For this review, take the finished solid that the model builds, in its own axes (mm). Face numbers are marked on the shaded views. A direction names the side the tool comes from. Coordinates: 2 decimals unless noted, no trailing zeros. Order: outer loops, then holes, each group sorted by start corner. A loop starts at its lowest first (then second) coordinate and runs counter-clockwise, first axis right, second up. Notation, with made-up numbers: (85.25, 70.5) -> (123.25, 70.5) arc R37 cw to (123.25, 109.5) -> close; hole circle Ø2 at (42.25, 24). An arc over 180 degrees is marked (long way). Write item = value, one per line. Start each with the question number.
1) Consider section A-A on x = -48. Give the boundary of the cut face in (y, z), and give its area (3 significant figures).
2) Consider section D-D on y = 59. Give the boundary of the cut face in (x, z).
3) Consider section B-B on y = 0. Give the boundary of the cut face in (x, z).
4) Draft analysis for pull direction Y (two halves, no side actions). For the marked faces 1, 2 and 3, state which applies: +Y half, -Y half, draft (parallel to the pull), parting line (faces both ways), or undercut.
5) Machinability: for the marked faces 4 and 5, which of the approach directions +Z, -Z, +X, -X, +Y, -Y give a long, thin tool a straight path to every point of the face, cutting with its end or side? Answer none if there is none.
6) Consider section C-C on z = 13.75. Give the boundary of the cut face in (x, y).
7) Insertion check: pin 1 Ø3 at (x, z) = (-5.5, 11.5) entering from -Y; pin 2 Ø1.5 at (x, z) = (2.5, 16.5) entering from +Y; pin 3 Ø3 at (y, z) = (67.5, 17.5) entering from -X. Each pin has a flat end and moves straight along its axis. Give the tip position at first contact, or say it passes through.
8) Wall thickness on probe 1 along X at (y, z) = (0, 13); probe 2 along Y at (x, z) = (0, 20.6); probe 3 along Z at (x, y) = (6.5, 47): over which ranges is each line inside the solid? List them lowest first. Write a range as [from, to].
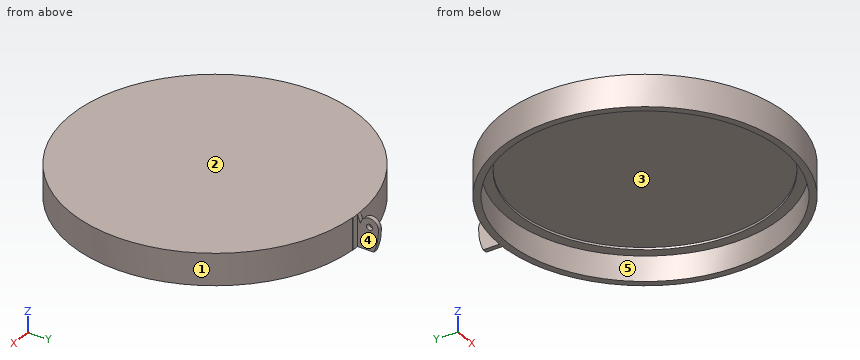
from build123d import *

# Parameters (mm, degrees)
SKETCH1_R                = 63.5
BOSS_EXTRUDE2_DEPTH      = 23
SHELL4_T                 = -3
SKETCH4_R                = 56.09702957
CUT_EXTRUDE1_DEPTH       = 22
BOSS_EXTRUDE6_DEPTH      = 1
BOSS_EXTRUDE6_DEPTH_BACK = 1
SKETCH8_R                = 1.3
BOSS_EXTRUDE7_REACH      = 145.843
BOSS_EXTRUDE7_END_RADIUS = 63.5
SKETCH9_W                = 5
SKETCH9_H                = 23
SKETCH11_R               = 63.5
CUT_EXTRUDE2_DEPTH       = 9
SKETCH12_W               = 19.480164653
SKETCH12_H               = 12.222333769
CUT_EXTRUDE3_DEPTH       = 13
BOSS_EXTRUDE8_START      = -2
SKETCH13_R               = 63.5
BOSS_EXTRUDE8_DEPTH      = 2


with BuildPart() as part:
    # Sketch1 → Boss-Extrude2 (new body)
    with BuildSketch(Plane.XY):
        Circle(SKETCH1_R)
    extrude(amount=BOSS_EXTRUDE2_DEPTH)

    # Shell4
    shell4_openings = [part.faces().sort_by_distance(p)[0] for p in [
        (0, 0, 0),
    ]]
    offset(amount=SHELL4_T, openings=shell4_openings, kind=Kind.INTERSECTION)

    # Sketch4 → Cut-Extrude1 (cut)
    with BuildSketch(Plane(origin=(0, 0, 20), x_dir=(-1, 0, 0), z_dir=(0, 0, -1))):
        Circle(SKETCH4_R)
    extrude(amount=-CUT_EXTRUDE1_DEPTH, mode=Mode.SUBTRACT)



with BuildPart() as body_2:
    # Sketch8 → Boss-Extrude6 (new, two sides: drawn at the far end of the back side and taken through both)
    with BuildSketch(Plane(origin=(0, 0, 0), x_dir=(0, 0, -1), z_dir=(1, 0, 0)).offset(-BOSS_EXTRUDE6_DEPTH_BACK)):
        with BuildLine():
            Line((-23, 63.5), (0, 63.5))
            ThreePointArc((0, 63.5), (-8.388517362, 70.509736152), (-19.092759253, 72.728481295))
            ThreePointArc((-19.092759253, 72.728481295), (-23.009560108, 68.811680441), (-19.092759253, 64.894879586))
            ThreePointArc((-19.092759253, 64.894879586), (-21.050529465, 64.209064035), (-23, 63.5))
        make_face()
        with Locations((-19.092759253, 68.811680441)):
            Circle(SKETCH8_R, mode=Mode.SUBTRACT)
    extrude(amount=BOSS_EXTRUDE6_DEPTH + BOSS_EXTRUDE6_DEPTH_BACK)


with BuildPart() as part_1:
    add(part.part)

    add(body_2.part)  # Boss-Extrude7 merges body 2
    # Boss-Extrude7: up to this cylinder (the profile starts outside it)
    boss_extrude7_end = Plane(origin=(0, 0, 11.5), z_dir=(0, 0, -1)) * Cylinder(BOSS_EXTRUDE7_END_RADIUS, 419.686, mode=Mode.PRIVATE)
    # Sketch9 → Boss-Extrude7 (add, up to the surface)
    with BuildSketch(Plane.XZ.offset(-63.5), mode=Mode.PRIVATE) as boss_extrude7_sk1:
        with Locations((1.5, 11.5)):
            Rectangle(SKETCH9_W, SKETCH9_H)
    boss_extrude7_tool1 = extrude(boss_extrude7_sk1.sketch, amount=BOSS_EXTRUDE7_REACH, mode=Mode.PRIVATE) - boss_extrude7_end
    add(boss_extrude7_tool1.solids().sort_by_distance((1.5, 63.5, 11.5))[0])
    add(boss_extrude7_tool1.solids().sort_by_distance((1.5, 63.5, 11.5))[1])

    # Sketch11 → Cut-Extrude2 (cut)
    with BuildSketch(Plane(origin=(0, 0, 0), x_dir=(-1, 0, 0), z_dir=(0, 0, -1))):
        Circle(SKETCH11_R)
    extrude(amount=-CUT_EXTRUDE2_DEPTH, mode=Mode.SUBTRACT)

    # Sketch12 → Cut-Extrude3 (cut)
    with BuildSketch(Plane(origin=(0, 0, 9), x_dir=(-1, 0, 0), z_dir=(0, 0, -1))):
        with Locations((1.337314283, 69.052754799)):
            Rectangle(SKETCH12_W, SKETCH12_H)
    extrude(amount=CUT_EXTRUDE3_DEPTH, mode=Mode.SUBTRACT)

    # Sketch13 → Boss-Extrude8 (add)
    with BuildSketch(Plane.XY.offset(23).offset(BOSS_EXTRUDE8_START)):
        Circle(SKETCH13_R)
    extrude(amount=BOSS_EXTRUDE8_DEPTH)


solid = part_1.part
Answer sheet:
q1.outline = (-41.57, 9) -> (-36.83, 9) -> (-36.83, 20) -> (-29.03, 20) -> (-29.03, 21) -> (29.03, 21) -> (29.03, 20) -> (36.83, 20) -> (36.83, 9) -> (41.57, 9) -> (41.57, 23) -> (-41.57, 23) -> close
q1.area = 296 mm2
q2.outline = (-23.48, 9) -> (-13.39, 9) -> (-13.39, 20) -> (13.39, 20) -> (13.39, 9) -> (23.48, 9) -> (23.48, 23) -> (-23.48, 23) -> close
q3.outline = (-63.5, 9) -> (-60.5, 9) -> (-60.5, 20) -> (-56.1, 20) -> (-56.1, 21) -> (56.1, 21) -> (56.1, 20) -> (60.5, 20) -> (60.5, 9) -> (63.5, 9) -> (63.5, 23) -> (-63.5, 23) -> close
q4.face_1 = parting line
q4.face_2 = draft
q4.face_3 = undercut
q5.face_4 = +Z, -Z, +X, +Y
q5.face_5 = -Z
q6.outline = (-1, 63.49) arc R63.5 ccw (long way) to (4, 63.37) -> (4, 63.5) -> (1, 63.5) -> (1, 72.31) -> (-1, 72.31) -> close; hole circle Ø121 at (0, 0)
q7.pin_1 = -63.37
q7.pin_2 = 63.5
q7.pin_3 = -1
q8.probe_1 = [-63.5, -60.5], [60.5, 63.5]
q8.probe_2 = [-63.5, -56.1], [56.1, 64.37], [65.2, 72.43]
q8.probe_3 = [21, 23]
